Geometry check sheet. Reference: the model listing, model coordinates, mm. A direction names the side the tool comes from. Coordinates: 2 decimals unless noted, no trailing zeros. Write each loop counter-clockwise with the first axis right and the second up, starting at its lowest first coordinate (ties: lowest second). Pieces come first, ordered by that corner, then holes. Notation, with made-up numbers: (-29, -9.75) -> (22, -9.75) arc R16 ccw to (22, -1.75) -> close; hole circle Ø3 at (-29, -38.5). An arc over 180 degrees is marked (long way). One line per question, with ' | ' between items.
from build123d import *

# Parameters (mm, degrees)
F0_W     = 193
F0_H     = 111
F0_W_2   = 179
F0_H_2   = 97
F1_DEPTH = 2
F0_R     = 4
F0_R_2   = 2
F2_DEPTH = 4.5
F3_DEPTH = 5
F4_DEPTH = 11.85


with BuildPart() as f1:
    # F0 (on Top) → F1 (new body)
    with BuildSketch(Plane.XY):
        with Locations((38.2122632861, 15.2387920618)):
            Rectangle(F0_W, F0_H)
        with Locations((38.2122632861, 15.2387920618)):
            Rectangle(F0_W_2, F0_H_2, mode=Mode.SUBTRACT)
    extrude(amount=F1_DEPTH)

    # F0 (on Top) → F2 (join)
    with BuildSketch(Plane.XY):
        with BuildLine():
            Line((143.2122632861, 80.2387920618), (-66.7877367139, 80.2387920618))
            Line((-66.7877367139, 80.2387920618), (-66.7877367139, -49.7612079382))
            Line((-66.7877367139, -49.7612079382), (-28.393488025, -49.7612079382))
            ThreePointArc((-28.393488025, -49.7612079382), (-27.393488025, -43.1154566271), (-21.7477367139, -46.7612079382))
            ThreePointArc((-21.7477367139, -46.7612079382), (-22.1019854028, -48.4069592493), (-23.1019854028, -49.7612079382))
            Line((-23.1019854028, -49.7612079382), (104.606511975, -49.7612079382))
            ThreePointArc((104.606511975, -49.7612079382), (105.606511975, -43.1154566271), (111.2522632861, -46.7612079382))
            ThreePointArc((111.2522632861, -46.7612079382), (110.8980145972, -48.4069592493), (109.8980145972, -49.7612079382))
            Line((109.8980145972, -49.7612079382), (143.2122632861, -49.7612079382))
            Line((143.2122632861, -49.7612079382), (143.2122632861, 80.2387920618))
        make_face()
        with Locations((38.2122632861, 15.2387920618)):
            Rectangle(F0_W, F0_H, mode=Mode.SUBTRACT)
        with Locations((-25.7477367139, 75.2387920618)):
            Circle(F0_R, mode=Mode.SUBTRACT)
        with Locations((107.2522632861, 75.2387920618)):
            Circle(F0_R, mode=Mode.SUBTRACT)
        with Locations((-25.7477367139, 75.2387920618)):
            Circle(F0_R)
        with Locations((-25.7477367139, 75.2387920618)):
            Circle(F0_R_2, mode=Mode.SUBTRACT)
        with Locations((107.2522632861, 75.2387920618)):
            Circle(F0_R)
        with Locations((107.2522632861, 75.2387920618)):
            Circle(F0_R_2, mode=Mode.SUBTRACT)
        with BuildLine():
            ThreePointArc((-21.7477367139, -46.7612079382), (-27.393488025, -43.1154566271), (-28.393488025, -49.7612079382))
            Line((-28.393488025, -49.7612079382), (-23.1019854028, -49.7612079382))
            ThreePointArc((-23.1019854028, -49.7612079382), (-22.1019854028, -48.4069592493), (-21.7477367139, -46.7612079382))
        make_face()
        with Locations((-25.7477367139, -46.7612079382)):
            Circle(F0_R_2, mode=Mode.SUBTRACT)
        with BuildLine():
            Line((104.606511975, -49.7612079382), (109.8980145972, -49.7612079382))
            ThreePointArc((109.8980145972, -49.7612079382), (110.8980145972, -48.4069592493), (111.2522632861, -46.7612079382))
            ThreePointArc((111.2522632861, -46.7612079382), (105.606511975, -43.1154566271), (104.606511975, -49.7612079382))
        make_face()
        with Locations((107.2522632861, -46.7612079382)):
            Circle(F0_R_2, mode=Mode.SUBTRACT)
    extrude(amount=F2_DEPTH)

    # F0 (on Top) → F3 (cut)
    with BuildSketch(Plane.XY):
        with Locations((-25.7477367139, 75.2387920618)):
            Circle(F0_R_2)
        with Locations((107.2522632861, 75.2387920618)):
            Circle(F0_R_2)
        with Locations((107.2522632861, -46.7612079382)):
            Circle(F0_R_2)
        with Locations((-25.7477367139, -46.7612079382)):
            Circle(F0_R_2)
    extrude(amount=-F3_DEPTH, mode=Mode.SUBTRACT)

    # F0 (on Top) → F4 (join)
    with BuildSketch(Plane.XY):
        with Locations((-25.7477367139, 75.2387920618)):
            Circle(F0_R)
        with Locations((-25.7477367139, 75.2387920618)):
            Circle(F0_R_2, mode=Mode.SUBTRACT)
        with BuildLine():
            Line((104.606511975, -49.7612079382), (109.8980145972, -49.7612079382))
            ThreePointArc((109.8980145972, -49.7612079382), (110.8980145972, -48.4069592493), (111.2522632861, -46.7612079382))
            ThreePointArc((111.2522632861, -46.7612079382), (105.606511975, -43.1154566271), (104.606511975, -49.7612079382))
        make_face()
        with Locations((107.2522632861, -46.7612079382)):
            Circle(F0_R_2, mode=Mode.SUBTRACT)
        with BuildLine():
            ThreePointArc((104.606511975, -49.7612079382), (107.2522632861, -50.7612079382), (109.8980145972, -49.7612079382))
            Line((109.8980145972, -49.7612079382), (104.606511975, -49.7612079382))
        make_face()
        with BuildLine():
            ThreePointArc((-21.7477367139, -46.7612079382), (-27.393488025, -43.1154566271), (-28.393488025, -49.7612079382))
            Line((-28.393488025, -49.7612079382), (-23.1019854028, -49.7612079382))
            ThreePointArc((-23.1019854028, -49.7612079382), (-22.1019854028, -48.4069592493), (-21.7477367139, -46.7612079382))
        make_face()
        with Locations((-25.7477367139, -46.7612079382)):
            Circle(F0_R_2, mode=Mode.SUBTRACT)
        with BuildLine():
            Line((-23.1019854028, -49.7612079382), (-28.393488025, -49.7612079382))
            ThreePointArc((-28.393488025, -49.7612079382), (-25.7477367139, -50.7612079382), (-23.1019854028, -49.7612079382))
        make_face()
        with Locations((107.2522632861, 75.2387920618)):
            Circle(F0_R)
        with Locations((107.2522632861, 75.2387920618)):
            Circle(F0_R_2, mode=Mode.SUBTRACT)
    extrude(amount=F4_DEPTH)


solid = f1.part
1. Mould release check, pull along Y, two halves, no side actions. Record for faces 1 (the face through (-66.788, 16, 2)), 2 (the face through (126, -49.761, 2)), 3 (the face through (31, -34, 2)): released by +Y, released by -Y, zero draft, split by the parting line, or undercut.
Worked answers:
face 1: zero draft | face 2: released by -Y | face 3: undercut
2. Material ranges on line 1 (X direction, y = 48, z = 3.75); line 2 (Y direction, x = -8, z = 0.75); line 3 (Y direction, x = -27, z = 10.75), recorded low to high. Write a range as from..to.
Worked answers:
line 1: -66.79..-58.29, 134.71..143.21 | line 2: -49.76..-33.26, 63.74..80.24 | line 3: -50.56..-48.32, -45.2..-42.96, 71.44..73.68, 76.8..79.04
3. Go/stop test with flat-tipped pins: P1, Ø2.5, axis at x = -25.75, y = -46.76, coming from the +Z side; P2, Ø4.5, axis at x = 107.25, y = -46.76, coming from the +Z side; P3, Ø1.3, axis at x = -42.5, z = 2, coming from the -Y side. Record where each tip stops, or that it passes through.
Worked answers:
P1: through | P2: z = 11.85 | P3: y = -49.76
4. Cross-section at A-A on y = -22. Record the boundary of the cut face in (x, z), and give its area (4 significant figures).
Worked answers:
outline: (-66.79, 0) -> (-51.29, 0) -> (-51.29, 2) -> (-58.29, 2) -> (-58.29, 4.5) -> (-66.79, 4.5) -> close; (127.71, 0) -> (143.21, 0) -> (143.21, 4.5) -> (134.71, 4.5) -> (134.71, 2) -> (127.71, 2) -> close | area: 104.5 mm²
5. Tool access check on faces 4 (the face through (105.665, 74.022, 5.842)), 5 (the face through (40, -49.761, 2)), 6 (the face through (106.7, 79.2, 8.1)). Record the directions out of +Z, -Z, +X, -X, +Y, -Y that give a thin tool (end or side, any length) a straight path to the whole face; none if there is none.
Worked answers:
face 4: +Z, -Z | face 5: +Z, -Z, -Y | face 6: +Z
6. Cross-section at B-B on x = 79. Record the boundary of the cut face in (y, z), and give its area (4 significant figures).
Worked answers:
outline: (-49.76, 0) -> (-33.26, 0) -> (-33.26, 2) -> (-40.26, 2) -> (-40.26, 4.5) -> (-49.76, 4.5) -> close; (63.74, 0) -> (80.24, 0) -> (80.24, 4.5) -> (70.74, 4.5) -> (70.74, 2) -> (63.74, 2) -> close | area: 113.5 mm²
7. Cross-section at C-C on z = 8.5. Record the boundary of the cut face in (x, y), and give its area (3 significant figures).
Worked answers:
outline: circle Ø8 at (-25.75, -46.76); circle Ø8 at (-25.75, 75.24); circle Ø8 at (107.25, -46.76); circle Ø8 at (107.25, 75.24); hole circle Ø4 at (-25.75, -46.76); hole circle Ø4 at (-25.75, 75.24); hole circle Ø4 at (107.25, -46.76); hole circle Ø4 at (107.25, 75.24) | area: 151 mm²
